For this review, take the finished solid that the model builds, in its own axes (mm). A direction names the side the tool comes from. Give positions to 0.01 mm unless a question says otherwise; leave off trailing zeros. Write each loop counter-clockwise with the first axis right and the second up, starting at its lowest first coordinate (ties: lowest second). Pieces come first, ordered by that corner, then holes. Notation, with made-up numbers: M 29.5,56 L 61.5,56 A20 ccw 61.5,94 Z; hole C 1,77 d2. An arc over 180 degrees is marked long. Write item = value, one per line.
Autodesk Inventor part; units mm, degrees
ref_plane "YZ Plane" through (0, 0, 0) normal (1, 0, 0) x (0, 1, 0)
ref_plane "XZ Plane" through (0, 0, 0) normal (0, 1, 0) x (-1, 0, 0)
ref_plane "XY Plane" through (0, 0, 0) normal (0, 0, 1) x (1, 0, 0)
sketch "スケッチ1" plane through (0, 0, 0) normal (0, 0, 1) x (1, 0, 0)
  line L0 (-59.5, -15) -> (59.5, -15) construction
  line L1 (59.5, -15) -> (59.5, 15) construction
  line L2 (59.5, 15) -> (-59.5, 15) construction
  line L3 (-59.5, 15) -> (-59.5, -15) construction
  line L4 (-59.5, -15) -> (59.5, 15) construction
  line L5 (59.5, -15) -> (-59.5, 15) construction
  line L6 (-59.5, 12.1) -> (-59.5, 15)
  line L7 (-59.5, 15) -> (59.5, 15)
  line L8 (59.5, 15) -> (59.5, 12.1)
  line L9 (-59.5, -12.1) -> (-59.5, -15)
  line L10 (59.5, -15) -> (59.5, -12.1)
  line L11 (-59.5, 10) -> (-62.5, 10)
  line L12 (-62.5, 10) -> (-62.5, -10)
  line L13 (-62.5, -10) -> (-59.5, -10)
  arc A0 (-59.5, 10) -> (-59.5, 12.1) centre (-59.5, 11.05) ccw
  line L14 (0, 0) -> (0, 15) construction
  line L15 (0, 0) -> (-59.5, 0) construction
  arc A1 (-59.5, -12.1) -> (-59.5, -10) centre (-59.5, -11.05) ccw
  line L16 (59.5, 10) -> (62.5, 10)
  line L17 (62.5, 10) -> (62.5, -10)
  line L18 (62.5, -10) -> (59.5, -10)
  arc A2 (59.5, 12.1) -> (59.5, 10) centre (59.5, 11.05) ccw
  arc A3 (59.5, -10) -> (59.5, -12.1) centre (59.5, -11.05) ccw
  line L19 (-59.5, -15) -> (-19.5, -18)
  line L20 (-19.5, -18) -> (19.5, -18)
  line L21 (19.5, -18) -> (59.5, -15)
  line L22 (-19.5, -10) -> (19.5, -10) construction
  line L23 (19.5, -10) -> (19.5, -15) construction
  line L24 (19.5, -15) -> (-19.5, -15) construction
  line L25 (-19.5, -15) -> (-19.5, -10) construction
  line L26 (19.55, -9.95) -> (-19.55, -9.95)
  line L27 (-19.55, -9.95) -> (-19.55, -15.05)
  line L28 (-19.55, -15.05) -> (19.55, -15.05)
  line L29 (19.55, -15.05) -> (19.55, -9.95)
  circle A4 centre (-18.5, -9.95) radius 1.05
  circle A5 centre (-18.5, -15.05) radius 1.05
  circle A6 centre (18.5, -9.95) radius 1.05
  circle A7 centre (18.5, -15.05) radius 1.05
  dimension "d9" = 2.1
  dimension "d0" = 119
  dimension "d1" = 30
  dimension "d2" = 1.05
  dimension "d3" = 20
  dimension "d4" = 3
  dimension "d5" = 5
  dimension "d6" = 0.05
  dimension "d7" = 39
  dimension "d8" = 3
extrude "押し出し1" add sketch "スケッチ1" along normal blind 5
sketch "スケッチ2" plane through (0, 0, 5) normal (0, 0, 1) x (1, 0, 0)
  line L0 (59.5, 12.1) -> (59.5, 15)
  line L1 (-59.5, 15) -> (-59.5, 12.1)
  line L2 (65.6261, 13.972) -> (59.5, 13.972)
  line L3 (59.5, 13.972) -> (59.5, -16.1)
  line L4 (59.5, -16.1) -> (65.6261, -16.1)
  line L5 (65.6261, -16.1) -> (65.6261, 13.972)
  line L6 (-65.8886, -16.1) -> (-59.5, -16.1)
  line L7 (-59.5, -16.1) -> (-59.5, 18.3327)
  line L8 (-59.5, 18.3327) -> (-65.8886, 18.3327)
  line L9 (-65.8886, 18.3327) -> (-65.8886, -16.1)
  point P0 (0, 0)
extrude "押し出し2" cut sketch "スケッチ2" against normal blind 2.5
sketch "スケッチ8" plane through (0, 0, 5) normal (0, 0, 1) x (1, 0, 0)
  line L0 (59.5, 15) -> (-59.5, 15)
  line L1 (-59.5, 10) -> (-59.5, -10)
  line L2 (-59.5, -15) -> (-19.5, -18)
  line L3 (17.45, -15.05) -> (-17.45, -15.05)
  arc A0 (-19.55, -15.05) -> (-17.45, -15.05) centre (-18.5, -15.05) ccw
  line L4 (-19.55, -15.05) -> (-19.55, -9.95)
  arc A1 (-17.45, -9.95) -> (-19.55, -9.95) centre (-18.5, -9.95) ccw
  line L5 (-17.45, -9.95) -> (17.45, -9.95)
  arc A2 (19.55, -9.95) -> (17.45, -9.95) centre (18.5, -9.95) ccw
  line L6 (19.55, -9.95) -> (19.55, -15.05)
  arc A3 (17.45, -15.05) -> (19.55, -15.05) centre (18.5, -15.05) ccw
  line L7 (-55.5, 12) -> (-22.5, 12) construction
  line L8 (-22.5, 12) -> (-22.5, -13.7638) construction
  line L9 (-22.5, -13.7638) -> (-55.5, -11.2888) construction
  line L10 (-55.5, -11.2888) -> (-55.5, 12) construction
  line L11 (17.5013, -10) -> (-17.5013, -10) construction
  arc A4 (-17.5013, -10) -> (-19.5, -9.95) centre (-18.5, -9.95) ccw construction
  line L12 (-19.5, -9.95) -> (-19.5, -15.05) construction
  arc A5 (-19.5, -15.05) -> (-17.5013, -15) centre (-18.5, -15.05) ccw construction
  line L13 (-17.5013, -15) -> (17.5013, -15) construction
  arc A6 (17.5013, -15) -> (19.5, -15.05) centre (18.5, -15.05) ccw construction
  line L14 (19.5, -15.05) -> (19.5, -9.95) construction
  arc A7 (19.5, -9.95) -> (17.5013, -10) centre (18.5, -9.95) ccw construction
  line L15 (-17.5, 12) -> (17.5, 12)
  line L16 (17.5, 12) -> (17.5, -5)
  line L17 (17.5, -5) -> (-17.5, -5)
  line L18 (-17.5, -5) -> (-17.5, 12)
  line L19 (0, 0) -> (0, 15) construction
  line L20 (-22.5, 12) -> (-55.5, -11.2888) construction
  line L21 (-55.5, 12) -> (-26.8358, 12)
  line L22 (-26.8358, 12) -> (-55.5, -8.2289)
  line L23 (-55.5, -8.2289) -> (-55.5, 12)
  line L24 (-51.5807, -11.5827) -> (-22.5, -13.7638)
  line L25 (-22.5, -13.7638) -> (-22.5, 8.9401)
  line L26 (-22.5, 8.9401) -> (-51.5807, -11.5827)
  line L27 (55.5, 12) -> (22.5, 12) construction
  line L28 (22.5, 12) -> (22.5, -13.7638) construction
  line L29 (22.5, -13.7638) -> (55.5, -11.2888) construction
  line L30 (55.5, -11.2888) -> (55.5, 12) construction
  line L31 (22.5, 12) -> (55.5, -11.2888) construction
  line L32 (55.5, 12) -> (26.8358, 12)
  line L33 (26.8358, 12) -> (55.5, -8.2289)
  line L34 (55.5, -8.2289) -> (55.5, 12)
  line L35 (51.5807, -11.5827) -> (22.5, -13.7638)
  line L36 (22.5, -13.7638) -> (22.5, 8.9401)
  line L37 (22.5, 8.9401) -> (51.5807, -11.5827)
  dimension "d51" = 4
  dimension "d52" = 3
  dimension "d53" = 0.05
  dimension "d54" = 3
  dimension "d55" = 4
  dimension "d56" = 5
  dimension "d57" = 5
  dimension "d58" = 5
extrude "押し出し6" cut sketch "スケッチ8" against normal blind 10 contours L15 L16 L17 L18 | L21 L22 L23 | L26 L25 L24 | L34 L33 L32 | L35 L36 L37
fillet "フィレット4" radius 2 12 edges at (-55.5, 12, 2.5) (-55.5, -8.2289, 2.5) (-26.8358, 12, 2.5) (-22.5, 8.9401, 2.5) (-51.5807, -11.5827, 2.5) (-22.5, -13.7638, 2.5) (22.5, 8.9401, 2.5) (26.8358, 12, 2.5) (55.5, -8.2289, 2.5) (55.5, 12, 2.5) (22.5, -13.7638, 2.5) (51.5807, -11.5827, 2.5)
fillet "フィレット4" radius 5 4 edges at (-17.5, -5, 2.5) (-17.5, 12, 2.5) (17.5, 12, 2.5) (17.5, -5, 2.5)
properties part number "コックピット_サブフレーム_1_6" material "アセタール樹脂、黒"
1. We need section A-A, the plane x = -42. Write out the cut boundary in (y, z).
Responses:
outline = M -16.31,0 L -12.3,0 L -12.3,5 L -16.31,5 Z; M -4.82,0 L 1.3,0 L 1.3,5 L -4.82,5 Z; M 12,0 L 15,0 L 15,5 L 12,5 Z
2. For line 1 along Y through (x, z) = (13, 4.75); line 2 along X through (y, z) = (-0.5, 1.15); line 3 along X through (y, z) = (-9.5, 4.7), list the stretches that pass through material, from the lowest coordinate up. Write a range as from..to.
Responses:
line_1 = -18..-15.05, -9.95..-4.97, 11.97..15
line_2 = -62.5..-55.5, -44.55..-35.88, -22.5..-17.47, 17.47..22.5, 35.88..44.55, 55.5..62.5
line_3 = -59.5..-47.81, -22.5..-19.45, -17.55..17.55, 19.45..22.5, 47.81..59.5
3. We need section B-B, the plane z = 3.6. Count the separate pieces of the cut face and the enclosed holes in it, then the cut area to 3 significant figures.
Responses:
separate_pieces = 1
enclosed_holes = 6
area = 1,820 mm2
4. Machinability: for faces 5 (the face through (16.07, -3.5, 2.46)), 6 (the face through (-59.5, 0, 4)), 7 (the face through (-61, 10, 1)), which of the approach directions +Z, -Z, +X, -X, +Y, -Y give a long, thin tool a straight path to every point of the face, cutting with its end or side? Answer none if there is none.
Responses:
face_5 = +Z, -Z
face_6 = +Z, -X, +Y, -Y
face_7 = +Z, -Z, -X, +Y
5. Insertion check: P1, Ø0.9, axis at y = -14, z = 3.5, coming from the -X side; P2, Ø1, axis at x = -36.5, z = 3.5, coming from the -Y side; P3, Ø1.2, axis at x = -61.5, z = 1, coming from the +Y side; P4, Ø8, axis at x = -26, y = 4.5, coming from the +Z side. Each pin has a flat end and moves straight along its axis. Give the tip position at first contact, or say it passes through.
Responses:
P1 = -59.5
P2 = -16.76
P3 = 10
P4 = 5
6. The part is to be moulded in two halves that separate along X. For faces 1 (the face through (-59.5, 14, 2)), 2 (the face through (0, -9.95, 2)), 3 (the face through (-16, -3.57, 2.46)), 4 (the face through (-61, -10, 1)), say which applies: +X half, -X half, draft (parallel to the pull), parting line (faces both ways), or undercut.
Responses:
face_1 = -X half
face_2 = undercut
face_3 = undercut
face_4 = draft
